from build123d import *

# Parameters (mm, degrees)
SKETCH2_R           = 2.25
BOSS_EXTRUDE1_DEPTH = 3.175


with BuildPart() as part:
    # Sketch2 → Boss-Extrude1 (new body)
    with BuildSketch(Plane(origin=(0, 0, 0), x_dir=(1, 0, 0), z_dir=(0, 1, 0))):
        with BuildLine():
            Line((19.7, -88.2), (31.525, -88.2))
            ThreePointArc((31.525, -88.2), (35.060533906, -86.735533906), (36.525, -83.2))
            Line((36.525, -83.2), (36.525, -70.7))
            Line((36.525, -70.7), (44.7, 0))
            ThreePointArc((44.7, 0), (0, 44.7), (-44.7, 0))
            Line((-44.7, 0), (-19.7, 0))
            ThreePointArc((-19.7, 0), (0, 19.7), (19.7, 0))
            Line((19.7, 0), (19.7, -88.2))
        make_face()
        with Locations((26.525, -80.975)):
            Circle(SKETCH2_R, mode=Mode.SUBTRACT)
        with Locations((26.525, -55.975)):
            Circle(SKETCH2_R, mode=Mode.SUBTRACT)
        with Locations((-17.67766953, 17.67766953)):
            Circle(SKETCH2_R, mode=Mode.SUBTRACT)
        with Locations((17.67766953, 17.67766953)):
            Circle(SKETCH2_R, mode=Mode.SUBTRACT)
    extrude(amount=BOSS_EXTRUDE1_DEPTH)


solid = part.part
Check sheet for the modelled part. Datum: model origin and axes. Units: mm. A direction names the side the tool comes from. Give positions to 0.01 mm unless a question says otherwise; leave off trailing zeros. Write each loop counter-clockwise with the first axis right and the second up, starting at its lowest first coordinate (ties: lowest second). Pieces come first, ordered by that corner, then holes. Notation, with made-up numbers: M -28,17 L 25,17 A10 cw 25,22 Z; hole C 71.5,15 d8. An arc over 180 degrees is marked long. Use one line per item in the form item = value.
(1) Draft check along X on faces 1 (the cylindrical face through (0.98, 1.57, -44.69)), 2 (the cylindrical face through (-0.433, 1.565, -19.695)), 3 (the flat face through (40.555, 1.565, 35.845)). Enter one of: pulls with the +X half, pulls with the -X half, needs draft (parallel to the pull), parting line crosses it, or undercut.
Answer block:
face_1 = parting line crosses it
face_2 = undercut
face_3 = pulls with the +X half
(2) Material ranges on line 1 along Z through (x, y) = (27.5, 0.3); line 2 along X through (y, z) = (1.25, -8.5); line 3 along X through (y, z) = (0.4, -6), recorded low to high.
Answer block:
line_1 = -35.24 to 53.95, 58 to 78.95, 83 to 88.2
line_2 = -43.88 to -17.77, 17.77 to 43.88
line_3 = -44.3 to -18.76, 18.76 to 44.3
(3) Section check C-C on x = 0. Record the boundary of the cut face in (y, z) (3 decimals).
Answer block:
outline = M 0,-44.7 L 3.175,-44.7 L 3.175,-19.7 L 0,-19.7 Z
(4) Tool access check on faces 4 (the cylindrical face through (-16.64, 1.57, -15.68)), 5 (the flat face through (19.7, 2, 43)), 6 (the flat face through (36.525, 2, 77)). Record the directions out of +Z, -Z, +X, -X, +Y, -Y that give a thin tool (end or side, any length) a straight path to the whole face; none if there is none.
Answer block:
face_4 = +Y, -Y
face_5 = +Z, -X, +Y, -Y
face_6 = +Z, +X, +Y, -Y
(5) Section check A-A on x = 18. Record the boundary of the cut face in (y, z) (3 decimals).
Answer block:
outline = M 0,-40.916 L 3.175,-40.916 L 3.175,-19.904 L 0,-19.904 Z; M 0,-15.451 L 3.175,-15.451 L 3.175,-8.006 L 0,-8.006 Z
(6) Depth check by flat-ended pin: P1, Ø1, axis at x = -27, y = 1.5, coming from the +Z side; P2, Ø1, axis at y = 2, z = 77, coming from the +X side (3 decimals). Enter the tip coordinate at first touch or a pass-through.
Answer block:
P1 = 0
P2 = 36.525
(7) Section check D-D on z = 49.5. Record the boundary of the cut face in (x, y) (3 decimals), plus the area to 3 significant figures.
Answer block:
outline = M 19.7,0 L 38.976,0 L 38.976,3.175 L 19.7,3.175 Z
area = 61.2 mm2
(8) Section check B-B on y = 1.25. Record the boundary of the cut face in (x, z) (3 decimals).
Answer block:
outline = M -44.7,0 A44.7 ccw 44.7,0 L 36.525,70.7 L 36.525,83.2 A5 ccw 31.525,88.2 L 19.7,88.2 L 19.7,0 A19.7 cw -19.7,0 Z; hole C -17.678,-17.678 d4.5; hole C 17.678,-17.678 d4.5; hole C 26.525,55.975 d4.5; hole C 26.525,80.975 d4.5
